Build history of the part. All positions in model axes, mm. Round coordinates to 2 decimals unless told otherwise and drop trailing zeros. Loops run counter-clockwise (first coordinate to the right, second up) from the corner with the lowest first, then second, coordinate; pieces in that order, holes last. Notation, with made-up numbers: (59.5, 86) -> (97.5, 86) arc R24 ccw to (97.5, 116) -> close; hole circle Ø2 at (11.5, 54). An arc over 180 degrees is marked (long way). Put each result on its own line as item: value. Start each with the question number.
Item 1: Cut at C-C, the plane z = -10.5. List the corners of the cut face in (x, y), plus the area to 3 significant figures.
Item 2: Cut at B-B, the plane x = 6. List the corners of the cut face in (y, z), plus the area to 3 significant figures.
Item 3: Drill centre lines: probe 1 along X at (y, z) = (1.9, -7.5); probe 2 along Z at (x, y) = (47.5, 1.85); probe 3 along Z at (x, y) = (11, 0.35). Where is each one in solid material? Low to high. Write a range as [from, to].
Item 4: Cut at A-A, the plane y = 2.4. List the corners of the cut face in (x, z).
Item 5: Flat gauge pins, fed straight in: pin 1 Ø1.5 at (y, z) = (1, -1.5) entering from +X; pin 2 Ø1.5 at (x, y) = (8.5, 2) entering from -Z; pin 3 Ø1.5 at (x, y) = (24, 1.5) entering from +Z; pin 4 Ø1.5 at (x, y) = (48, 1.5) entering from -Z. Where does each tip first touch, or does it go through?
```python
from build123d import *

# Parameters (mm, degrees)
ESQUISSE1_W             = 50
ESQUISSE1_H             = 50
BOSS_EXTRU_1_DEPTH      = 3
ENL_V_MAT_EXTRU_1_DEPTH = 3


with BuildPart() as part:
    # Esquisse1 → Boss.-Extru.1 (new body)
    with BuildSketch(Plane(origin=(0, 0, 0), x_dir=(1, 0, 0), z_dir=(0, 1, 0))):
        with Locations((25, 25)):
            Rectangle(ESQUISSE1_W, ESQUISSE1_H)
    extrude(amount=BOSS_EXTRU_1_DEPTH)

    # Esquisse2 → Enlèv. mat.-Extru.1 (cut)
    with BuildSketch(Plane(origin=(0, 3, 0), x_dir=(1, 0, 0), z_dir=(0, 1, 0))):
        Polygon((0, 37.5), (3, 37.5), (3, 47), (12.5, 47), (12.5, 50), (0, 50), align=None)
        Polygon((0, 12.5), (3, 12.5), (3, 3), (12.5, 3), (12.5, 0), (0, 0), align=None)
        Polygon((50, 12.5), (47, 12.5), (47, 3), (37.5, 3), (37.5, 0), (50, 0), align=None)
        Polygon((37.5, 50), (37.5, 47), (47, 47), (47, 37.5), (50, 37.5), (50, 50), align=None)
    extrude(amount=-ENL_V_MAT_EXTRU_1_DEPTH, mode=Mode.SUBTRACT)


solid = part.part
```
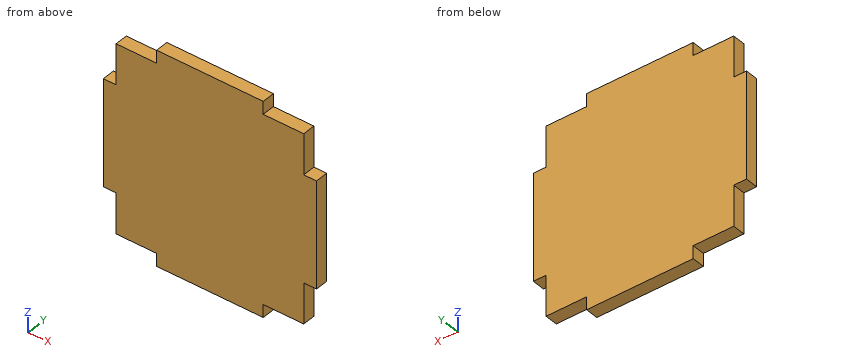
Reply:
1. outline: (3, 0) -> (47, 0) -> (47, 3) -> (3, 3) -> close
1. area: 132 mm^2
2. outline: (0, -47) -> (3, -47) -> (3, -3) -> (0, -3) -> close
2. area: 132 mm^2
3. probe 1: x = [3, 47]
3. probe 2: z = [-37.5, -12.5]
3. probe 3: z = [-47, -3]
4. outline: (0, -37.5) -> (3, -37.5) -> (3, -47) -> (12.5, -47) -> (12.5, -50) -> (37.5, -50) -> (37.5, -47) -> (47, -47) -> (47, -37.5) -> (50, -37.5) -> (50, -12.5) -> (47, -12.5) -> (47, -3) -> (37.5, -3) -> (37.5, 0) -> (12.5, 0) -> (12.5, -3) -> (3, -3) -> (3, -12.5) -> (0, -12.5) -> close
5. pin 1: stops at x = 37.5
5. pin 2: stops at z = -47
5. pin 3: stops at z = 0
5. pin 4: stops at z = -37.5
